Can you work these out from the model? Positions are in its coordinate system, mm. Coordinates: 2 decimals unless noted, no trailing zeros. Write each loop counter-clockwise with the first axis right and the second up, starting at its lowest first coordinate (ties: lowest second). Pieces come first, ordered by that corner, then holes. Notation, with made-up numbers: (69, 69.5) -> (106, 69.5) arc R9 ccw to (106, 86.5) -> close; hole circle Ø3 at (-2, 66.5). An arc over 180 degrees is marked (long way). Answer as CSV lines item,"result". Start each with the question number.
Autodesk Inventor part; units mm, degrees
ref_plane "YZ Plane" through (0, 0, 0) normal (1, 0, 0) x (0, 1, 0)
ref_plane "XZ Plane" through (0, 0, 0) normal (0, 1, 0) x (-1, 0, 0)
ref_plane "XY Plane" through (0, 0, 0) normal (0, 0, 1) x (1, 0, 0)
sketch "Sketch1" plane through (0, 0, 0) normal (0, 1, 0) x (-1, 0, 0)
  line L0 (-363.3, 419.1) -> (363.3, 419.1)
  line L1 (368.3, 414.1) -> (368.3, -414.1)
  line L2 (363.3, -419.1) -> (-363.3, -419.1)
  line L3 (-368.3, -414.1) -> (-368.3, 414.1)
  line L4 (-368.3, 419.1) -> (368.3, -419.1) construction
  line L5 (368.3, 419.1) -> (-368.3, -419.1) construction
  line L6 (303.3, 359.1) -> (-303.3, 359.1)
  line L7 (-308.3, 354.1) -> (-308.3, -354.1)
  line L8 (-303.3, -359.1) -> (303.3, -359.1)
  line L9 (308.3, -354.1) -> (308.3, 354.1)
  arc A0 (308.3, 354.1) -> (303.3, 359.1) centre (303.3, 354.1) ccw
  arc A1 (303.3, -359.1) -> (308.3, -354.1) centre (303.3, -354.1) ccw
  arc A2 (-303.3, 359.1) -> (-308.3, 354.1) centre (-303.3, 354.1) ccw
  arc A3 (-308.3, -354.1) -> (-303.3, -359.1) centre (-303.3, -354.1) ccw
  arc A4 (368.3, 414.1) -> (363.3, 419.1) centre (363.3, 414.1) ccw
  arc A5 (-363.3, 419.1) -> (-368.3, 414.1) centre (-363.3, 414.1) ccw
  arc A6 (-368.3, -414.1) -> (-363.3, -419.1) centre (-363.3, -414.1) ccw
  arc A7 (363.3, -419.1) -> (368.3, -414.1) centre (363.3, -414.1) ccw
  point P0 (0, 0)
  dimension "d0" = 736.6
  dimension "d1" = 838.2
  dimension "d2" = 60
  dimension "d4" = 5
extrude "Extrusion1" add sketch "Sketch1" along normal blind 5
sketch "Sketch2" plane through (0, 5, 0) normal (0, 1, 0) x (1, 0, 0)
  circle A0 centre (-334, 384.8) radius 6
  circle A1 centre (-250.5, 384.8) radius 6
  circle A2 centre (-167, 384.8) radius 6
  circle A3 centre (-83.5, 384.8) radius 6
  circle A4 centre (0, 384.8) radius 6
  circle A5 centre (83.5, 384.8) radius 6
  circle A6 centre (-334, 288.6) radius 6
  circle A7 centre (-334, 96.2) radius 6
  circle A8 centre (-334, -96.2) radius 6
  circle A9 centre (-334, -192.4) radius 6
  circle A10 centre (-334, -288.6) radius 6
  circle A11 centre (-334, -384.8) radius 6
  circle A12 centre (-334, 0) radius 6
  circle A13 centre (-334, 192.4) radius 6
  circle A14 centre (-250.5, -384.8) radius 6
  circle A15 centre (-167, -384.8) radius 6
  circle A16 centre (-83.5, -384.8) radius 6
  circle A17 centre (0, -384.8) radius 6
  circle A18 centre (83.5, -384.8) radius 6
  circle A19 centre (167, -384.8) radius 6
  circle A20 centre (250.5, -384.8) radius 6
  circle A21 centre (334, -384.8) radius 6
  circle A22 centre (334, -288.6) radius 6
  circle A23 centre (334, -192.4) radius 6
  circle A24 centre (334, -96.2) radius 6
  circle A25 centre (334, 0) radius 6
  circle A26 centre (334, 96.2) radius 6
  circle A27 centre (334, 192.4) radius 6
  circle A28 centre (334, 288.6) radius 6
  circle A29 centre (334, 384.8) radius 6
  circle A30 centre (167, 384.8) radius 6
  circle A31 centre (250.5, 384.8) radius 6
  point P0 (0, 0)
extrude "Extrusion2" cut sketch "Sketch2" against normal up to next contours A0 | A2 | A4 | A9 | A11 | A12 | A13 | A15 | A17 | A19 | A21 | A23 | A25 | A27 | A29 | A30
properties part number "H3NE-FF"
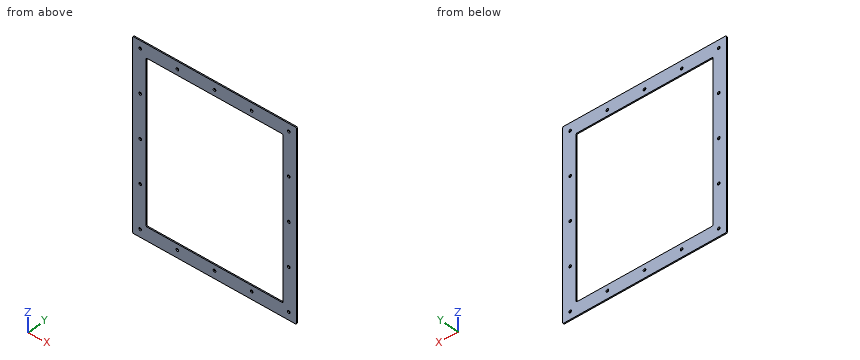
Q1. Imagine slicing it at A-A (y = 2.4). State how many separate pieces and enclosed holes the cut face has, then the cut area to 3 significant figures.
Q2. Imagine slicing it at B-B (z = 172.5). Write out the boundary of the cut face in (x, y), then the cut area to 3 significant figures.
Q3. I need wall thicknesses on L1, parallel to X at y = 1.7, z = -192.4; L2, parallel to X at y = 1.1, z = 384.8; L3, parallel to Z at x = -334, y = 2.35. Which ranges of each line are inside material? Lowest first, please.
Q4. Imagine slicing it at C-C (x = 211.5). Write out the boundary of the cut face in (y, z).
Entries:
1,separate pieces,"1"
1,enclosed holes,"17"
1,area,"173,000 mm2"
2,outline,"(-368.3, 0) -> (-308.3, 0) -> (-308.3, 5) -> (-368.3, 5) -> close; (308.3, 0) -> (368.3, 0) -> (368.3, 5) -> (308.3, 5) -> close"
2,area,"600 mm2"
3,L1,"-368.3 to -340, -328 to -308.3, 308.3 to 328, 340 to 368.3"
3,L2,"-368.3 to -340, -328 to -173, -161 to -6, 6 to 161, 173 to 328, 340 to 368.3"
3,L3,"-419.1 to -390.8, -378.8 to -198.4, -186.4 to -6, 6 to 186.4, 198.4 to 378.8, 390.8 to 419.1"
4,outline,"(0, -419.1) -> (5, -419.1) -> (5, -359.1) -> (0, -359.1) -> close; (0, 359.1) -> (5, 359.1) -> (5, 419.1) -> (0, 419.1) -> close"
